Source: three-view drawing plus pictorial views. Frame: mm from the lowest corner of the part. A direction names the side the tool comes from. Round coordinates to 2 decimals unless told otherwise and drop trailing zeros. Loops run counter-clockwise (first coordinate to the right, second up) from the corner with the lowest first, then second, coordinate; pieces in that order, holes last. Notation, with made-up numbers: M 27.25,-28.5 L 48.25,-28.5 A22 ccw 48.25,-17.5 Z; hole C 1,-23.75 d9. An arc over 180 degrees is marked long. Return JSON: item names as keys, results as strings. Group by question number.
1) Section B-B (z = 90). Output: boundary loops of the cut face in (x, y), plus the area to 3 significant figures.
2) Section D-D (z = 50). Output: boundary loops of the cut face in (x, y).
3) Section A-A (x = 90). Output: boundary loops of the cut face in (y, z).
4) Mould query, pull axis X, two halves, no side actions, for the marked faces 3, 4 and 5. Classes: +X half, -X half, draft (parallel to the pull), parting line (faces both ways), or undercut.
5) Material intervals for line 1 (X direction, y = 8.5, z = 50); line 2 (X direction, y = 24.5, z = 50); line 3 (X direction, y = 24.5, z = 67), sorted ascending. Write a range as from..to.
6) Contact query for flat-ended pins moving along their axis: P1, Ø5, axis at x = 11.5, y = 10, coming from the +Z side; P2, Ø1, axis at y = 18.5, z = 60, coming from the +X side; P3, Ø3, axis at x = 10, z = 50, coming from the +Y side; P4, Ø12, axis at y = 22, z = 33, coming from the +X side (3 decimals). Output: stop coordinate, or through.
7) Section C-C (y = 27.5). Output: boundary loops of the cut face in (x, z).
8) Access query for the marked faces 1 and 2. Directions: +Z, -Z, +X, -X, +Y, -Y. A direction counts if a zero-diameter tool reaches every point of the face in a straight line with its end or side. Return the directions, or none.
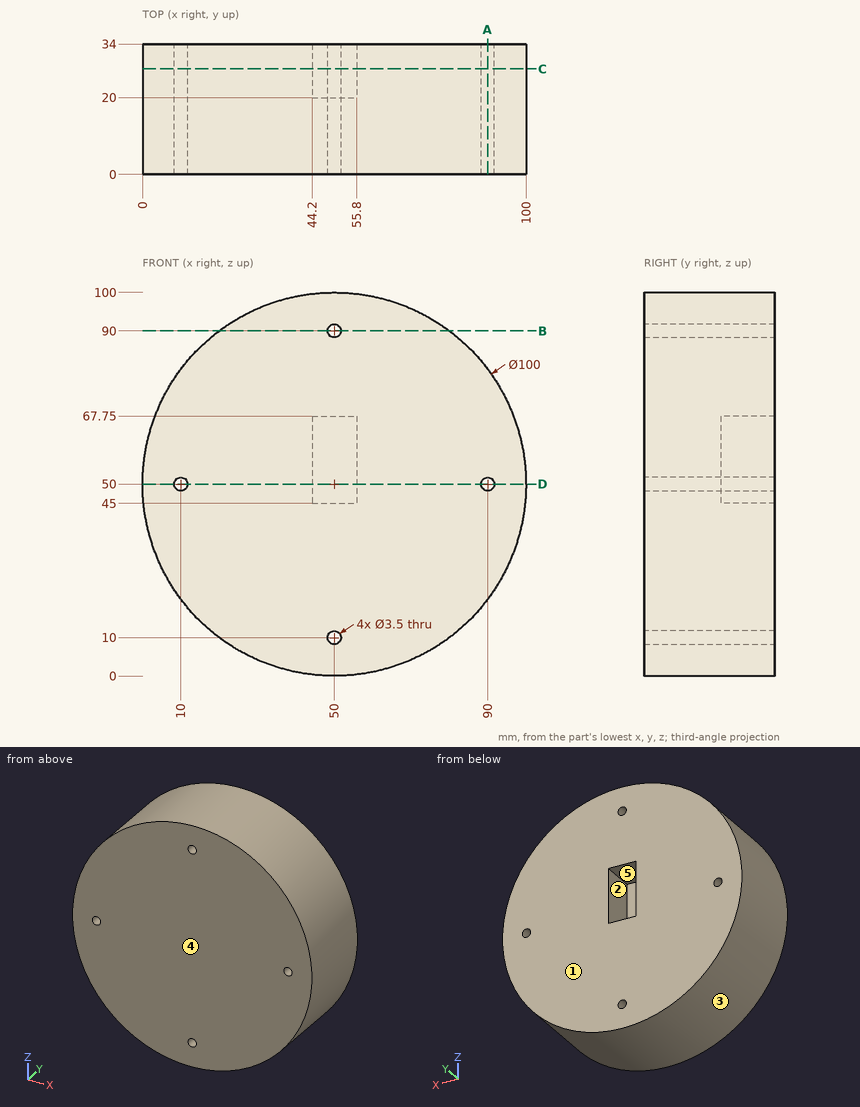
Returned:
{
 "1": {"outline": "M 20,0 L 48.25,0 L 48.25,34 L 20,34 Z; M 51.75,0 L 80,0 L 80,34 L 51.75,34 Z", "area": "1,920 mm^2"},
 "2": {"outline": "M 0,0 L 8.25,0 L 8.25,34 L 0,34 Z; M 11.75,0 L 88.25,0 L 88.25,34 L 55.8,34 L 55.8,20 L 44.2,20 L 44.2,34 L 11.75,34 Z; M 91.75,0 L 100,0 L 100,34 L 91.75,34 Z"},
 "3": {"outline": "M 0,20 L 34,20 L 34,48.25 L 0,48.25 Z; M 0,51.75 L 34,51.75 L 34,80 L 0,80 Z"},
 "4": {"face 3": "parting line", "face 4": "draft", "face 5": "undercut"},
 "5": {"line 1": "x = 0..8.25, 11.75..88.25, 91.75..100", "line 2": "x = 0..8.25, 11.75..44.2, 55.8..88.25, 91.75..100", "line 3": "x = 2.98..44.2, 55.8..97.02"},
 "6": {"P1": "stops at z = 84.7", "P2": "stops at x = 99.09", "P3": "passes through", "P4": "stops at x = 98.775"},
 "7": {"outline": "C 50,50 d100; hole C 10,50 d3.5; hole M 44.2,45 L 55.8,45 L 55.8,67.75 L 44.2,67.75 Z; hole C 50,10 d3.5; hole C 50,90 d3.5; hole C 90,50 d3.5"},
 "8": {"face 1": "+Z, -Z, +X, -X, +Y", "face 2": "+Y"}
}
